```python
from build123d import *

# Parameters (mm, degrees)
F0_R     = 10
F1_DEPTH = 20
F2_R     = 15
F3_DEPTH = 5


with BuildPart() as f1:
    # F0 (on Front) → F1 (new body)
    with BuildSketch(Plane.XZ):
        Circle(F0_R)
    extrude(amount=F1_DEPTH)

    # F2 (on face) → F3 (join)
    with BuildSketch(Plane.XZ.offset(20)):
        Circle(F2_R)
    extrude(amount=F3_DEPTH)

    # F4: F1 across face


with BuildPart() as f1_1:
    add(f1.part)
    add(f1.part.mirror(Plane(origin=(0, 0, 0), x_dir=(1, 0, 0), z_dir=(0, 1, 0))))


solid = f1_1.part
```
Verification items for the finished model (mm, model axes). A direction names the side the tool comes from. Round coordinates to 2 decimals unless told otherwise and drop trailing zeros. Write each loop counter-clockwise with the first axis right and the second up, starting at its lowest first coordinate (ties: lowest second). Pieces come first, ordered by that corner, then holes. Notation, with made-up numbers: (67, 31.5) - (120, 31.5) arc R36 ccw to (120, 66.5) - close; hole circle Ø8 at (37.25, 30.25). An arc over 180 degrees is marked (long way). Answer as a JSON object with one key per item and string values. Group by question number.
Q1. Section check A-A, the plane z = -10.75. Enter the section's corners in (x, y).
Q2. Go/stop test with flat-tipped pins: pin 1 Ø4 at (y, z) = (19, 10) entering from -X; pin 2 Ø8 at (x, y) = (-2, -9) entering from -Z; pin 3 Ø3 at (x, y) = (-5.5, -16.5) entering from +Z. Record where each tip stops, or that it passes through.
Q3. Thickness scan on line 1 (Y direction, x = -13, z = -2); line 2 (Z direction, x = -6.25, y = -7); line 3 (X direction, y = -0.5, z = 8.5). Record the ranges inside material, lowest first.
Q4. Section check C-C, the plane z = 0. Enter the section's corners in (x, y).
Q5. Tool access check on faces 1 (the cylindrical face through (-14.985, 22.465, 0.66)), 2 (the flat face through (3, -20, -10)). Record the directions out of +Z, -Z, +X, -X, +Y, -Y that give a thin tool (end or side, any length) a straight path to the whole face; none if there is none.
Q6. Mould release check, pull along Y, two halves, no side actions. Record for faces 3 (the cylindrical face through (-14.985, -22.465, 0.66)), 4 (the cylindrical face through (-2.17, -0.28, -9.76)), 5 (the flat face through (0, 25, 0)): released by +Y, released by -Y, zero draft, split by the parting line, or undercut.
Q7. Section check B-B, the plane x = 0. Enter the section's corners in (y, z), plus the area to 3 significant figures.
Found:
{
 "1": {"outline": "(-10.46, -25) - (10.46, -25) - (10.46, -20) - (-10.46, -20) - close; (-10.46, 20) - (10.46, 20) - (10.46, 25) - (-10.46, 25) - close"},
 "2": {"pin 1": "stops at x = -12.52", "pin 2": "stops at z = -10", "pin 3": "stops at z = 9.17"},
 "3": {"line 1": "y = -25 to -20, 20 to 25", "line 2": "z = -7.81 to 7.81", "line 3": "x = -5.27 to 5.27"},
 "4": {"outline": "(-15, -25) - (15, -25) - (15, -20) - (10, -20) - (10, 20) - (15, 20) - (15, 25) - (-15, 25) - (-15, 20) - (-10, 20) - (-10, -20) - (-15, -20) - close"},
 "5": {"face 1": "+Y, -Y", "face 2": "none"},
 "6": {"face 3": "zero draft", "face 4": "undercut", "face 5": "released by +Y"},
 "7": {"outline": "(-25, -15) - (-20, -15) - (-20, -10) - (20, -10) - (20, -15) - (25, -15) - (25, 15) - (20, 15) - (20, 10) - (-20, 10) - (-20, 15) - (-25, 15) - close", "area": "1,100 mm^2"}
}
